from build123d import *

# Parameters (mm, degrees)
F2_DEPTH = 12.7
F3_DEPTH = 6.35
F4_W     = 1.7614989947
F4_H     = 6.35
F5_DEPTH = 6.35
F7_DEPTH = 6.35


with BuildPart() as f1:
    # F0 (on Front) → F1 (revolve)
    with BuildSketch(Plane.XZ):
        Polygon((12.7, 9.4802887884), (6.35, 9.4802887884), (6.35, 34.8802887884), (0, 34.8802887884), (0, -5.9427527222), (12.7, -9.345707466), align=None)
        Polygon((0, -15.9197112116), (12.7, -15.9197112116), (0, -12.5167564678), align=None)
        Polygon((12.7, -15.9197112116), (12.7, -9.345707466), (0, -5.9427527222), (0, -12.5167564678), align=None)
    revolve(axis=Axis((0, 0, 9.4802887884), (0, 0, 1)))

    # F0 (on Front) → F2 (cut, symmetric)
    with BuildSketch(Plane.XZ):
        Polygon((-12.7, -15.9197112116), (0, -15.9197112116), (0, -12.5167564678), (-12.7, -9.1138017239), align=None)
        Polygon((0, -15.9197112116), (12.7, -15.9197112116), (0, -12.5167564678), align=None)
    extrude(amount=F2_DEPTH, both=True, mode=Mode.SUBTRACT)

    # F0 (on Front) → F3 (cut)
    with BuildSketch(Plane.XZ):
        Polygon((0, -12.5167564678), (0, -5.9427527222), (-11.0564990636, -2.980172727), (-12.7, -9.1138017239), align=None)
        Polygon((12.7, -15.9197112116), (12.7, -9.345707466), (0, -5.9427527222), (0, -12.5167564678), align=None)
        Polygon((-12.7, -9.1138017239), (-11.0564990636, -2.980172727), (-12.7, -2.5397979783), align=None)
    extrude(amount=-F3_DEPTH, mode=Mode.SUBTRACT)

    # F4 (on face) → F5 (cut)
    with BuildSketch(Plane(origin=(-3.1291891169, 0, -11.6782927709), x_dir=(0.9659258263, 0, -0.2588190451), z_dir=(-0.2588190451, 0, -0.9659258263))):
        with BuildLine():
            Line((-8.1469335398, 6.35), (3.5889137071, 6.35))
            Line((3.5889137071, 6.35), (14.6260834533, 6.35))
            add(Edge.make_bspline(
                [(3.2395749568, 12.7), (10.8305806211, 12.7), (14.6260834533, 6.35)],
                knots=[1.5707963268, 1.5707963268, 1.5707963268, 2.6058232788, 2.6058232788, 2.6058232788], degree=2, weights=[1, 0.8070072037, 0.8683475024]))
            add(Edge.make_bspline(
                [(-8.1469335398, 6.35), (-4.3514307076, 12.7), (3.2395749568, 12.7)],
                knots=[0.5357693748, 0.5357693748, 0.5357693748, 1.5707963268, 1.5707963268, 1.5707963268], degree=2, weights=[0.8683475024, 0.8070072037, 1]))
        make_face()
        with BuildLine():
            Line((-8.1469335398, 12.7), (-8.1469335398, 6.35))
            add(Edge.make_bspline(
                [(-8.1469335398, 6.35), (-4.3514307076, 12.7), (3.2395749568, 12.7)],
                knots=[0.5357693748, 0.5357693748, 0.5357693748, 1.5707963268, 1.5707963268, 1.5707963268], degree=2, weights=[0.8683475024, 0.8070072037, 1]))
            Line((3.2395749568, 12.7), (-8.1469335398, 12.7))
        make_face()
        with Locations((-9.0276830371, 9.525)):
            Rectangle(F4_W, F4_H)
    extrude(amount=-F5_DEPTH, mode=Mode.SUBTRACT)

    # F6 (on face) → F7 (cut)
    with BuildSketch(Plane.XZ.offset(6.35)):
        with BuildLine():
            Line((-4.3968861542, -8.0516125007), (-7.4637006527, -7.2298620325))
            ThreePointArc((-7.4637006527, -7.2298620325), (-6.3411686376, -9.1741445159), (-4.3968861542, -8.0516125007))
        make_face()
        with BuildLine():
            ThreePointArc((-4.3427934035, -7.6407372666), (-5.7230830733, -6.0668185492), (-7.4637006527, -7.2298620325))
            Line((-7.4637006527, -7.2298620325), (-4.3968861542, -8.0516125007))
            ThreePointArc((-4.3968861542, -8.0516125007), (-4.356374686, -7.8479475968), (-4.3427934035, -7.6407372666))
        make_face()
        with BuildLine():
            Line((6.3983008804, -10.9441741488), (9.4651153788, -11.765924617))
            ThreePointArc((9.4651153788, -11.765924617), (9.505626847, -11.562259713), (9.5192081296, -11.3550493829))
            ThreePointArc((9.5192081296, -11.3550493829), (8.1389184597, -9.7811306655), (6.3983008804, -10.9441741488))
        make_face()
        with BuildLine():
            ThreePointArc((6.3983008804, -10.9441741488), (7.5208328955, -12.8884566321), (9.4651153788, -11.765924617))
            Line((9.4651153788, -11.765924617), (6.3983008804, -10.9441741488))
        make_face()
    extrude(amount=-F7_DEPTH, mode=Mode.SUBTRACT)


solid = f1.part
For this review, take the finished solid that the model builds, in its own axes (mm). A direction names the side the tool comes from. Round coordinates to 2 decimals unless told otherwise and drop trailing zeros. Write each loop counter-clockwise with the first axis right and the second up, starting at its lowest first coordinate (ties: lowest second). Pieces come first, ordered by that corner, then holes. Notation, with made-up numbers: (-31, -13.75) -> (19, -13.75) arc R14 cw to (19, 8.25) -> close; hole circle Ø6 at (72.25, 66.25). An arc over 180 degrees is marked (long way). Use CSV: the item, a comma, the result in double quotes.
(1) Consider section B-B, the plane z = 8. Give the boundary of the cut face in (x, y).
Computed values:
outline,"circle Ø25.4 at (0, 0)"
(2) Clearance check with flat-ended pins moving along their axes: P1, Ø1, axis at y = -4, z = -9.5, coming from the -X side; P2, Ø1.5, axis at y = 9.5, z = -2.5, coming from the -X side; P3, Ø2, axis at y = 3, z = 0.5, coming from the -X side. State where each tip first meets the part, or that it passes through.
Computed values:
P1,"x = -12.19"
P2,"x = -9.2"
P3,"x = -12.54"
(3) To check wall thickness, follow L1, parallel to Z at x = 0, y = -2.75; L2, parallel to Y at x = -8, z = -7; L3, parallel to Y at x = -8.75, z = -4. State the ranges of each line that lie inside material, in increasing order. Write a range as [from, to].
Computed values:
L1,"[-12.52, 34.88]"
L2,"[-6.35, 0], [6.35, 9.86]"
L3,"[-6.35, 0], [6.35, 9.2]"
(4) For faces 4 (the face through (3, 6, 9.48)), 5 (the face through (-0.154, -8.864, -5.901)), 6 (the face through (0, 6.35, -9)), 7 (the face through (6.827, 10.709, -0.22)), list the 3-axis set-ups (+Z, -Z, +X, -X, +Y, -Y) from which the entire face can be reached by the end or side of a thin tool; tool diameter is ignored.
Computed values:
face 4,"+Z"
face 5,"-Z, -X, -Y"
face 6,"-Z, -X"
face 7,"+Z, -Z"
(5) Draft analysis for pull direction Y (two halves, no side actions). For faces 1 (the face through (0, -6.35, -9)), 2 (the face through (-1.38, -6.2, 22.36)), 3 (the face through (0, 0, -9)), state which applies: +Y half, -Y half, draft (parallel to the pull), parting line (faces both ways), or undercut.
Computed values:
face 1,"-Y half"
face 2,"parting line"
face 3,"undercut"
(6) Consider section D-D, the plane z = 32. Give the boundary of the cut face in (x, y), plus the area to 3 significant figures.
Computed values:
outline,"circle Ø12.7 at (0, 0)"
area,"127 mm²"
(7) Consider section A-A, the plane y = -3.25. Give the boundary of the cut face in (x, z) (1 decimal).
Computed values:
outline,"(-12.3, -9.2) -> (12.3, -15.8) -> (12.3, 9.5) -> (5.5, 9.5) -> (5.5, 34.9) -> (-5.5, 34.9) -> (-5.5, 9.5) -> (-12.3, 9.5) -> close; hole circle Ø3.2 at (-5.9, -7.6); hole circle Ø3.2 at (7.9, -11.4)"
(8) Consider section C-C, the plane y = -0.5. Give the boundary of the cut face in (x, z) (1 decimal).
Computed values:
outline,"(-12.7, -9.1) -> (12.7, -15.9) -> (12.7, 9.5) -> (6.3, 9.5) -> (6.3, 34.9) -> (-6.3, 34.9) -> (-6.3, 9.5) -> (-12.7, 9.5) -> close; hole circle Ø3.2 at (-5.9, -7.6); hole circle Ø3.2 at (7.9, -11.4)"
